The listing builds one solid part. Answer for the finished solid, in the listing's coordinates (mm). Face numbers are marked on the shaded views. A direction names the side the tool comes from. Coordinates: 2 decimals unless noted, no trailing zeros. Loops run counter-clockwise (first coordinate to the right, second up) from the corner with the lowest first, then second, coordinate; pieces in that order, holes last. Notation, with made-up numbers: M -19,-25 L 38,-25 A34 cw 38,11 Z; hole C 35,-1.75 d5. An arc over 180 degrees is marked long. Answer as a JSON object with one key per item and string values. Group by question number.
1. Determine the mould class of the marked faces 3, 4 and 5 for opening direction X: released by +X, released by -X, zero draft, split by the parting line, or undercut.
2. A cutting plane is placed at C-C on y = 5. Give the vertices of the cut face in (x, z).
3. Given pin 1 (2 mm diameter, centred on y = 4.5, z = 0, fed in from -X); pin 2 (3 mm diameter, centred on x = -1, y = -1, fed in from -Z); pin 3 (1.5 mm diameter, centred on y = -1, z = -2, fed in from -X); pin 4 (1.5 mm diameter, centred on x = -1.5, z = -1.5, fed in from +Y), each flat-ended and moving along its own axis, determine where each tip first touches the part or whether it passes through.
4. A cutting plane is placed at B-B on z = -0.3. Give the vertices of the cut face in (x, y), and give its area (3 significant figures).
5. For the marked faces 1 and 2, determine the directions among +Z, -Z, +X, -X, +Y, -Y from which every point of the face is accessible in a straight line to the end or side of a thin tool.
6. A cutting plane is placed at A-A on x = 0. Give the vertices of the cut face in (y, z), and give its area (3 significant figures).
7. Straight lines are drawn through the part: L1, parallel to Y at x = 0, z = -1.4; L2, parallel to Z at x = 4, y = 3.25; L3, parallel to Y at x = -2.25, z = -1. For each, find the intervals that lie inside material, in ascending order.
8. A cutting plane is placed at D-D on x = -4.75. Give the vertices of the cut face in (y, z), and give its area (3 significant figures).
Autodesk Inventor part; units mm, degrees
ref_plane "YZ Plane" through (0, 0, 0) normal (1, 0, 0) x (0, 1, 0)
ref_plane "XZ Plane" through (0, 0, 0) normal (0, 1, 0) x (-1, 0, 0)
ref_plane "XY Plane" through (0, 0, 0) normal (0, 0, 1) x (1, 0, 0)
sketch "Szkic1" plane through (0, 0, 0) normal (0, 0, 1) x (1, 0, 0)
  circle A0 centre (0, 0) radius 3
  circle A1 centre (0, 0) radius 4
  circle A2 centre (0, 0) radius 6
  dimension "d0" = 6
  dimension "d1" = 8
  dimension "d2" = 12
extrude "Wyciągnięcie proste1" add sketch "Szkic1" along normal blind 1 contours A1 | A2
extrude "Wyciągnięcie proste2" add sketch "Szkic1" against normal blind 3 contours A1
sketch "Szkic2" plane through (0, 0, 1) normal (0, 0, 1) x (1, 0, 0)
  circle A0 centre (0, 0) radius 4
  line L0 (4, 0) -> (5.899, 1.0964)
  circle A1 centre (0, 0) radius 6
  line L1 (4, 0) -> (5.9306, -1.1146)
  line L2 (4, 0) -> (6, 0) construction
  circle A2 centre (0, 0) radius 6 construction
  circle A3 centre (0, 0) radius 6 construction
  circle A4 centre (0, 0) radius 3 construction
  point P0 (5.899, -1.0964)
  dimension "d7" = 60
  dimension "d8" = 30
extrude "Wyciągnięcie proste3" cut sketch "Szkic2" against normal blind 10 contours L0 A1 L1 picked at (5.2847, 0.6099)
chamfer "Faza1" distance 0.4 angle 45 1 edges at (-4, 0, -3)
chamfer "Faza2" distance 0.5 angle 45 1 edges at (-3, 0, -3)
equation "\"d8\" = 0.5 * d7"
properties part number "tuleja_TUF106040"
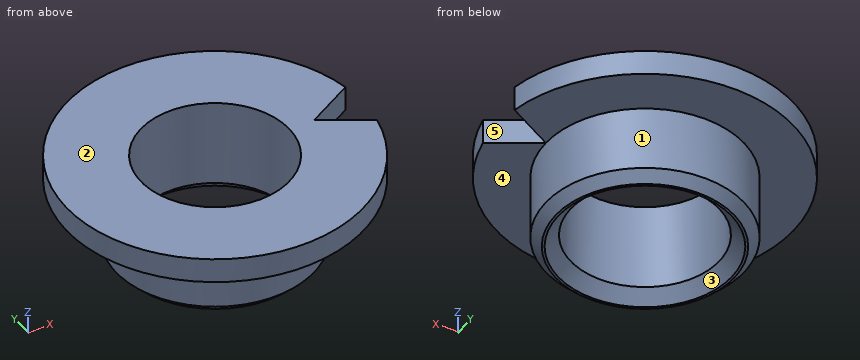
From the geometry:
{
 "1": {"face 3": "undercut", "face 4": "zero draft", "face 5": "released by +X"},
 "2": {"outline": "M -3.32,0 L 3.32,0 L 3.32,1 L -3.32,1 Z"},
 "3": {"pin 1": "stops at x = -4.87", "pin 2": "passes through", "pin 3": "stops at x = -3.99", "pin 4": "stops at y = 3.93"},
 "4": {"outline": "C 0,0 d8; hole C 0,0 d6", "area": "22.0 mm²"},
 "5": {"face 1": "-Z", "face 2": "+Z, +X, -X, +Y, -Y"},
 "6": {"outline": "M -6,0 L -4,0 L -4,-2.6 L -3.6,-3 L -3.5,-3 L -3,-2.5 L -3,1 L -6,1 Z; M 3,-2.5 L 3.5,-3 L 3.6,-3 L 4,-2.6 L 4,0 L 6,0 L 6,1 L 3,1 Z", "area": "11.6 mm²"},
 "7": {"L1": "y = -4 to -3, 3 to 4", "L2": "z = 0 to 1", "L3": "y = -3.31 to -1.98, 1.98 to 3.31"},
 "8": {"outline": "M -3.67,0 L 3.67,0 L 3.67,1 L -3.67,1 Z", "area": "7.33 mm²"}
}
